The drawing under review shows one solid part. Ordinate dimensions are in mm from its lowest x, y, z. A direction names the side the tool comes from. Coordinates: 2 decimals unless noted, no trailing zeros. Order: outer loops, then holes, each group sorted by start corner. A loop starts at its lowest first (then second) coordinate and runs counter-clockwise, first axis right, second up. Notation, with made-up numbers: (-33, -18) - (-17, -18) arc R34 ccw to (-17, 14) - close; hole circle Ø6 at (45, 70.25). An arc over 180 degrees is marked (long way). Write item = value, one per line. Start each with the question number.
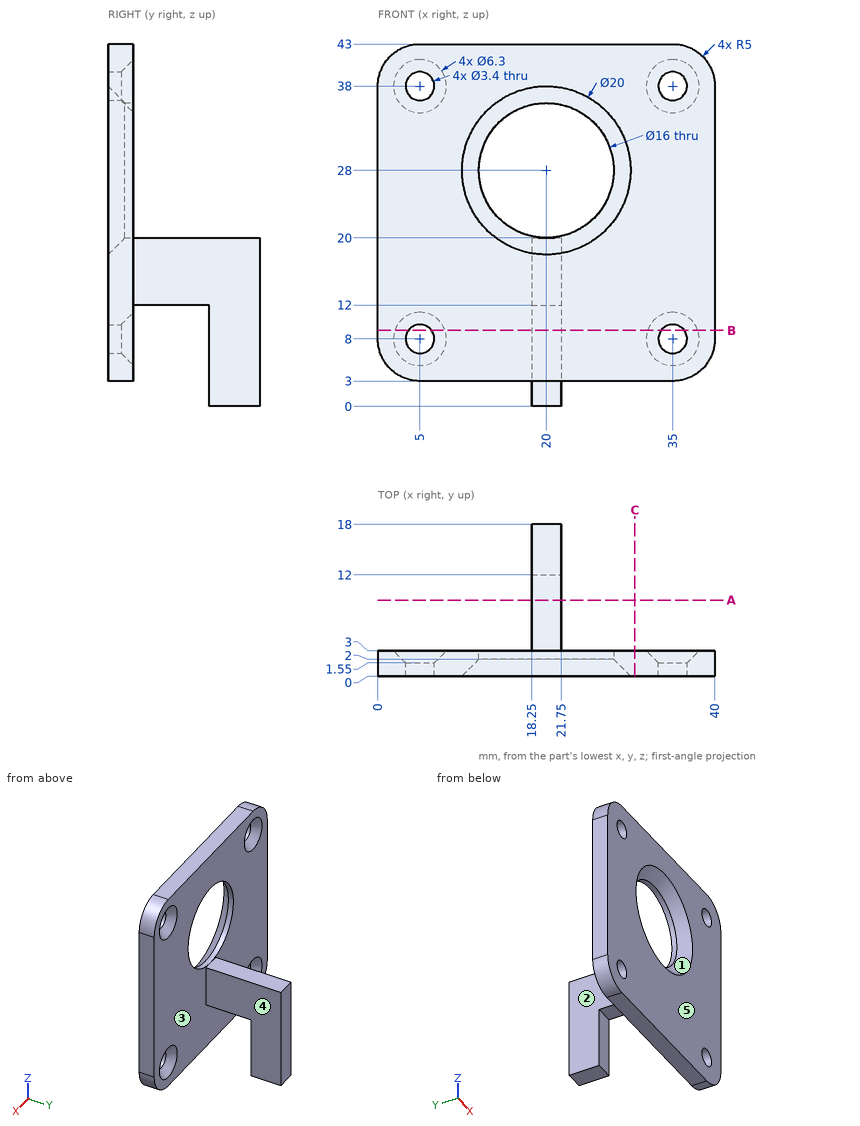
Item 1: Add section B-B on z = 9. State how many separate pieces and enclosed holes the cut face has, plus the area to 3 significant figures.
Item 2: For P1, Ø0.9, axis at x = 18.5, y = 1, coming from the -Z side; P2, Ø1.5, axis at x = 31.5, z = 35, coming from the +Y side; P3, Ø5.5, axis at x = 35, z = 38, coming from the +Y side, all flat-tipped, find the tip position at first contact; note any pin that passes through.
Item 3: Mouldability with a two-part tool opening along X and no side actions: class the marked faces 1, 2 and 3 as +X half, -X half, draft (parallel to the pull), parting line (faces both ways), or undercut.
Item 4: For line 1 (X direction, y = 0.8, z = 8); line 2 (Z direction, x = 35, y = 0.6); line 3 (Z direction, x = 20, y = 2.35), list the stretches that pass through material, from the lowest coordinate up.
Item 5: Add section C-C on x = 30.5. Give the boundary of the cut face in (y, z), plus the area to 3 significant figures.
Item 6: Add section A-A on y = 9. Give the boundary of the cut face in (x, z).
Item 7: For the marked faces 4 and 5, list the 3-axis set-ups (+Z, -Z, +X, -X, +Y, -Y) from which the entire face can be reached by the end or side of a thin tool; tool diameter is ignored.
Worked out:
q1.separate_pieces = 4
q1.enclosed_holes = 0
q1.area = 120 mm2
q2.P1 = 3
q2.P2 = 3
q2.P3 = 2.6
q3.face_1 = undercut
q3.face_2 = -X half
q3.face_3 = draft
q4.line_1 = 0 to 3.3, 6.7 to 33.3, 36.7 to 40
q4.line_2 = 3 to 6.3, 9.7 to 36.3, 39.7 to 43
q4.line_3 = 3 to 20, 36 to 43
q5.outline = (0, 3) - (3, 3) - (3, 43) - (0, 43) - close
q5.area = 120 mm2
q6.outline = (18.25, 12) - (21.75, 12) - (21.75, 20) - (18.25, 20) - close
q7.face_4 = +Z, -Z, +X, +Y
q7.face_5 = +Z, -Z, +X, -X, -Y
